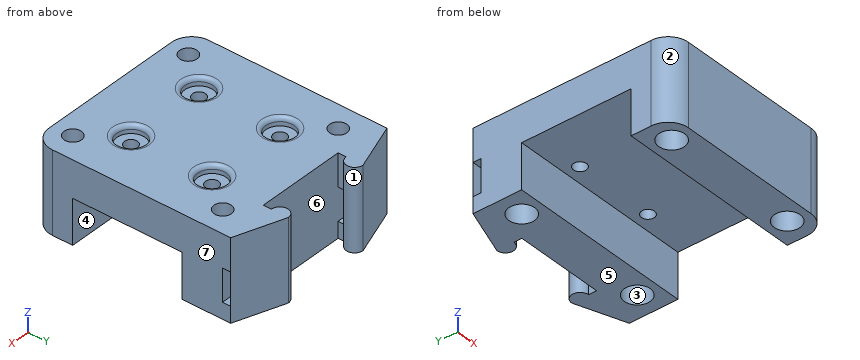
```python
from build123d import *

# Parameters (mm, degrees)
SKETCH1_W               = 46
SKETCH1_H               = 47
BOSS_EXTRUDE1_DEPTH     = 9
SKETCH2_R               = 1.6
CUT_EXTRUDE1_DEPTH      = 10
SKETCH3_W               = 46
SKETCH3_H               = 10
BOSS_EXTRUDE2_DEPTH     = 11
SKETCH4_R               = 2.15
CUT_EXTRUDE2_DEPTH      = 10
CUT_EXTRUDE2_DEPTH_BACK = 12
BOSS_EXTRUDE5_DEPTH     = 20
SKETCH8_W               = 8
SKETCH8_H               = 2
CUT_EXTRUDE3_DEPTH      = 24
CUT_EXTRUDE3_DEPTH_BACK = 24
SKETCH9_R               = 3.5
CUT_EXTRUDE4_DEPTH      = 2
FILLET1_R               = 1
FILLET2_R               = 5
SKETCH10_R              = 3.2
CUT_EXTRUDE5_DEPTH      = 13


with BuildPart() as part:
    # Sketch1 → Boss-Extrude1 (new body)
    with BuildSketch(Plane.XY):
        Rectangle(SKETCH1_W, SKETCH1_H)
    extrude(amount=BOSS_EXTRUDE1_DEPTH)

    # Sketch2 → Cut-Extrude1 (cut)
    with BuildSketch(Plane.XY.offset(9)):
        with Locations((-10, 10)):
            Circle(SKETCH2_R)
        with Locations((10, 10)):
            Circle(SKETCH2_R)
        with Locations((-10, -10)):
            Circle(SKETCH2_R)
        with Locations((10, -10)):
            Circle(SKETCH2_R)
    extrude(amount=-CUT_EXTRUDE1_DEPTH, mode=Mode.SUBTRACT)

    # Sketch3 → Boss-Extrude2 (add)
    with BuildSketch(Plane.XY):
        with Locations((0, 18.5)):
            Rectangle(SKETCH3_W, SKETCH3_H)
        with Locations((0, -18.5)):
            Rectangle(SKETCH3_W, SKETCH3_H)
    extrude(amount=-BOSS_EXTRUDE2_DEPTH)

    # Sketch4 → Cut-Extrude2 (cut, two sides)
    with BuildSketch(Plane.XY) as cut_extrude2_sk:
        with Locations((-17, 18.5)):
            Circle(SKETCH4_R)
        with Locations((17, 18.5)):
            Circle(SKETCH4_R)
        with Locations((-17, -18.5)):
            Circle(SKETCH4_R)
        with Locations((17, -18.5)):
            Circle(SKETCH4_R)
    extrude(amount=CUT_EXTRUDE2_DEPTH, mode=Mode.SUBTRACT)
    extrude(cut_extrude2_sk.sketch, amount=-CUT_EXTRUDE2_DEPTH_BACK, mode=Mode.SUBTRACT)

    # Sketch7 → Boss-Extrude5 (add)
    with BuildSketch(Plane(origin=(0, 0, -11), x_dir=(-1, 0, 0), z_dir=(0, 0, -1))):
        with BuildLine():
            Line((-23, 23.5), (-11, 23.5))
            Line((-11, 23.5), (-11, 25.5))
            ThreePointArc((-11, 25.5), (-8.920338159, 27.579661841), (-11, 29.659323681))
            Line((-11, 29.659323681), (-23, 25.5))
            Line((-23, 25.5), (-23, 23.5))
        make_face()
        with BuildLine():
            Line((23, 23.5), (11, 23.5))
            Line((11, 23.5), (11, 25.5))
            ThreePointArc((11, 25.5), (8.920338159, 27.579661841), (11, 29.659323681))
            Line((11, 29.659323681), (23, 25.5))
            Line((23, 25.5), (23, 23.5))
        make_face()
    extrude(amount=-BOSS_EXTRUDE5_DEPTH)

    # Sketch8 → Cut-Extrude3 (cut, two sides)
    with BuildSketch(Plane(origin=(0, 0, 0), x_dir=(0, 0, -1), z_dir=(1, 0, 0))) as cut_extrude3_sk:
        with Locations((3, 24.5)):
            Rectangle(SKETCH8_W, SKETCH8_H)
    extrude(amount=CUT_EXTRUDE3_DEPTH, mode=Mode.SUBTRACT)
    extrude(cut_extrude3_sk.sketch, amount=-CUT_EXTRUDE3_DEPTH_BACK, mode=Mode.SUBTRACT)

    # Sketch9 → Cut-Extrude4 (cut)
    with BuildSketch(Plane.XY.offset(9)):
        with Locations((-10, 10)):
            Circle(SKETCH9_R)
        with Locations((10, 10)):
            Circle(SKETCH9_R)
        with Locations((10, -10)):
            Circle(SKETCH9_R)
        with Locations((-10, -10)):
            Circle(SKETCH9_R)
    extrude(amount=-CUT_EXTRUDE4_DEPTH, mode=Mode.SUBTRACT)

    # Fillet1
    fillet1_edges = [part.edges().sort_by_distance(p)[0] for p in [
        (-13.5, -10, 9),
        (6.5, -10, 9),
        (6.5, 10, 9),
        (-13.5, 10, 9),
    ]]
    fillet(fillet1_edges, radius=FILLET1_R)

    # Fillet2
    fillet2_edges = [part.edges().sort_by_distance(p)[0] for p in [
        (23, -23.5, -1),
        (-23, -23.5, -1),
    ]]
    fillet(fillet2_edges, radius=FILLET2_R)

    # Sketch10 → Cut-Extrude5 (cut)
    with BuildSketch(Plane(origin=(0, 0, -11), x_dir=(-1, 0, 0), z_dir=(0, 0, -1))):
        with Locations((-17, -18.5)):
            Circle(SKETCH10_R)
        with Locations((17, -18.5)):
            Circle(SKETCH10_R)
        with Locations((17, 18.5)):
            Circle(SKETCH10_R)
        with Locations((-17, 18.5)):
            Circle(SKETCH10_R)
    extrude(amount=-CUT_EXTRUDE5_DEPTH, mode=Mode.SUBTRACT)


solid = part.part
```
CAD build for the part. Positions are in the model's coordinates, mm. Face numbers are marked on the shaded views. A direction names the side the tool comes from. Coordinates: 2 decimals unless noted, no trailing zeros. Order: outer loops, then holes, each group sorted by start corner. A loop starts at its lowest first (then second) coordinate and runs counter-clockwise, first axis right, second up. Notation, with made-up numbers: (47.25, 18.5) -> (79.25, 18.5) arc R13 ccw to (79.25, 22.5) -> close; hole circle Ø1 at (35, 25). An arc over 180 degrees is marked (long way). Use one line per item in the form item = value. Start each with the question number.
1) Tool access for the marked faces 1, 2, 3 and 4: list every direction of +Z, -Z, +X, -X, +Y, -Y with a clear straight run to the whole face (end or side of a thin tool).
2) Band-saw the part on D-D on x = -2. Give the cut face in (y, z), then the cut area to 3 significant figures.
3) Band-saw the part on A-A on z = -0.75. Give the cut face in (x, y), then the cut area to 3 significant figures.
4) Pull direction Z, two halves, no side cores. Call the marked faces 5, 6 and 7: +Z half, -Z half, draft (parallel to the pull), parting line (faces both ways), or undercut.
5) Band-saw the part on C-C on y = -10. Give the cut face in (x, z).
6) Drop flat-ended pins along their axis: pin 1 (5.5 mm diameter, centred on x = 17, y = -18.5, fed in from -Z); pin 2 (3.5 mm diameter, centred on x = 17, y = 18.5, fed in from -Z); pin 3 (7.5 mm diameter, centred on x = 17, y = -18.5, fed in from -Z); pin 4 (5.5 mm diameter, centred on x = 10, y = -10, fed in from +Z). Give the stop position or say it passes through.
7) Band-saw the part on B-B on z = -7.75. Give the cut face in (x, y), then the cut area to 3 significant figures.
8) Drill centre lines: L1, parallel to Y at x = 11, z = -3; L2, parallel to X at y = -18.5, z = 7.5; L3, parallel to Y at x = 10, z = -4.25. Where is each one in solid material? Low to high. Write a range as [from, to].
Entries:
q1.face_1 = +Z, -Z
q1.face_2 = +Z, -Z, -X, -Y
q1.face_3 = -Z
q1.face_4 = -Z, +X, -X
q2.outline = (-23.5, -11) -> (-13.5, -11) -> (-13.5, 0) -> (13.5, 0) -> (13.5, -11) -> (23.5, -11) -> (23.5, 9) -> (-23.5, 9) -> close
q2.area = 643 mm2
q3.outline = (-23, -18.5) arc R5 ccw to (-18, -23.5) -> (18, -23.5) arc R5 ccw to (23, -18.5) -> (23, -13.5) -> (-23, -13.5) -> close; (-23, 13.5) -> (23, 13.5) -> (23, 23.5) -> (-23, 23.5) -> close; (-23, 25.5) -> (-11, 25.5) arc R2.08 ccw to (-11, 29.66) -> close; (11, 25.5) -> (23, 25.5) -> (11, 29.66) arc R2.08 ccw to start; hole circle Ø6.4 at (-17, -18.5); hole circle Ø6.4 at (-17, 18.5); hole circle Ø6.4 at (17, -18.5); hole circle Ø6.4 at (17, 18.5)
q3.area = 844 mm2
q4.face_5 = -Z half
q4.face_6 = undercut
q4.face_7 = draft
q5.outline = (-23, 0) -> (-11.6, 0) -> (-11.6, 7) -> (-13.5, 7) -> (-13.5, 8) arc R1 ccw to (-14.5, 9) -> (-23, 9) -> close; (-8.4, 0) -> (8.4, 0) -> (8.4, 7) -> (6.5, 7) -> (6.5, 8) arc R1 ccw to (5.5, 9) -> (-5.5, 9) arc R1 ccw to (-6.5, 8) -> (-6.5, 7) -> (-8.4, 7) -> close; (11.6, 0) -> (23, 0) -> (23, 9) -> (14.5, 9) arc R1 ccw to (13.5, 8) -> (13.5, 7) -> (11.6, 7) -> close
q6.pin_1 = 2
q6.pin_2 = through
q6.pin_3 = -11
q6.pin_4 = 7
q7.outline = (-23, -18.5) arc R5 ccw to (-18, -23.5) -> (18, -23.5) arc R5 ccw to (23, -18.5) -> (23, -13.5) -> (-23, -13.5) -> close; (-23, 13.5) -> (23, 13.5) -> (23, 25.5) -> (11, 29.66) arc R2.08 ccw to (11, 25.5) -> (11, 23.5) -> (-11, 23.5) -> (-11, 25.5) arc R2.08 ccw to (-11, 29.66) -> (-23, 25.5) -> close; hole circle Ø6.4 at (-17, -18.5); hole circle Ø6.4 at (-17, 18.5); hole circle Ø6.4 at (17, -18.5); hole circle Ø6.4 at (17, 18.5)
q7.area = 892 mm2
q8.L1 = [-23.5, -13.5], [13.5, 23.5], [25.5, 29.66]
q8.L2 = [-23, -19.15], [-14.85, 14.85], [19.15, 23]
q8.L3 = [-23.5, -13.5], [13.5, 23.5], [25.76, 29.4]
